Answer from the drawing. Dimensions are ordinates in mm from the lowest x, y and z of the part. A direction names the side the tool comes from. Coordinates: 2 decimals unless noted, no trailing zeros. Order: outer loops, then holes, each group sorted by start corner. A loop starts at its lowest first (then second) coordinate and runs counter-clockwise, first axis right, second up. Notation, with made-up numbers: (-4, 40.5) - (50, 40.5) arc R24 ccw to (50, 51.5) - close; hole circle Ø1 at (31.25, 54). An arc over 180 degrees is marked (long way). Use a Markdown table: item, result. Add a question column.
Item 1: Flat-ended cylindrical pins translate along their axes: P1, Ø5, axis at y = 40.5, z = 20, coming from the +X side; P2, Ø2, axis at y = 15, z = 28, coming from the +X side; P3, Ø6, axis at y = 39, z = 8.5, coming from the -X side. Find the tip coordinate at first contact, or state that the pin passes through.
Item 2: The part is cut by section A-A, the plane z = 47. Give the vertices of the cut face in (x, y), then the cut area to 3 significant figures.
Item 3: For the marked faces 1 and 2, determine the directions among +Z, -Z, +X, -X, +Y, -Y from which every point of the face is accessible in a straight line to the end or side of a thin tool.
Item 4: The part is cut by section D-D, the plane x = 32.5. Give the vertices of the cut face in (y, z).
Item 5: The part is cut by section C-C, the plane z = 25. Give the vertices of the cut face in (x, y), then the cut area to 3 significant figures.
Item 6: The part is cut by section B-B, the plane x = 24. Give the vertices of the cut face in (y, z).
Item 7: The mould has two halves that part along X. Classify the marked faces 3, 4, 5 and 6: released by +X, released by -X, zero draft, split by the parting line, or undercut.
Item 8: Find the intervals of material crossed by line 1 along Y through (x, z) = (24.5, 46); line 2 along X through (y, z) = (34, 19.5); line 3 along X through (y, z) = (14.5, 23.5) (3 decimals), in increasing order.
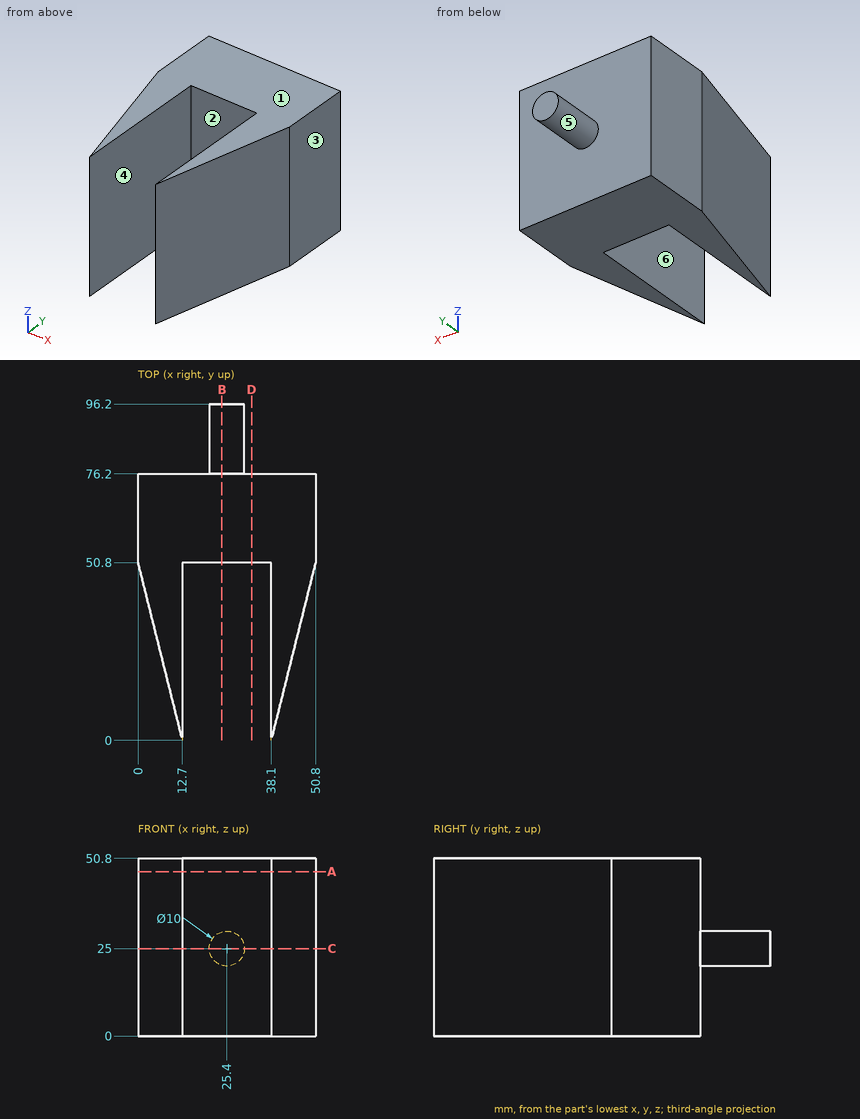
Solution:
| question | item | result |
|---|---|---|
| 1 | P1 | stops at x = 48.85 |
| 1 | P2 | stops at x = 42.1 |
| 1 | P3 | stops at x = 2.2 |
| 2 | outline | (0, 50.8) - (12.7, 0) - (12.7, 50.8) - (38.1, 50.8) - (38.1, 0) - (50.8, 50.8) - (50.8, 76.2) - (0, 76.2) - close |
| 2 | area | 1,940 mm2 |
| 3 | face 1 | +Z, +X, -X, +Y, -Y |
| 3 | face 2 | +Z, -Z, -Y |
| 4 | outline | (50.8, 0) - (76.2, 0) - (76.2, 50.8) - (50.8, 50.8) - close |
| 5 | outline | (0, 50.8) - (12.7, 0) - (12.7, 50.8) - (38.1, 50.8) - (38.1, 0) - (50.8, 50.8) - (50.8, 76.2) - (30.4, 76.2) - (30.4, 96.2) - (20.4, 96.2) - (20.4, 76.2) - (0, 76.2) - close |
| 5 | area | 2,140 mm2 |
| 6 | outline | (50.8, 0) - (76.2, 0) - (76.2, 20.2) - (96.2, 20.2) - (96.2, 29.8) - (76.2, 29.8) - (76.2, 50.8) - (50.8, 50.8) - close |
| 7 | face 3 | released by +X |
| 7 | face 4 | undercut |
| 7 | face 5 | split by the parting line |
| 7 | face 6 | undercut |
| 8 | line 1 | y = 50.8 to 76.2 |
| 8 | line 2 | x = 4.2 to 12.7, 38.1 to 46.6 |
| 8 | line 3 | x = 9.075 to 12.7, 38.1 to 41.725 |
